Could you check a few things on this model? Use its own coordinates, in mm. A direction names the side the tool comes from. Give positions to 0.01 mm unless a question says otherwise; leave off trailing zeros. Loops run counter-clockwise (first coordinate to the right, second up) from the corner with the lowest first, then second, coordinate; pieces in that order, holes last. Notation, with made-up numbers: (-40, 44) -> (13, 44) arc R28 ccw to (13, 83) -> close; hole circle Ø8 at (88, -9). An arc over 180 degrees is marked (long way). Write item = value, one per line. Start each with the question number.
1) I want a section at A-A (z = 2.5). List the corners of the cut face in (x, y) for me, and give its area (3 significant figures).
2) I want a section at B-B (y = 13.5). List the corners of the cut face in (x, z) for me.
3) On a 3-axis mill with a long thin cutter (end or side, diameter ignored), from which of +Z, -Z, +X, -X, +Y, -Y can I reach the whole of each face in a straight line? I mean faces 1 (the face through (3, 4, 2)), 2 (the face through (-0.434, 10.793, 4.452)), 3 (the face through (-4.815, 1.215, 0.075)), 4 (the face through (-3, 4, 2)), 5 (the face through (-4.8, 1.1, 2.5)). Say none if no direction works.
4) I need wall thicknesses on probe 1 along X at (y, z) = (10.75, 2.45); probe 2 along X at (y, z) = (4.75, 2.3); probe 3 along Y at (x, z) = (-2.75, 2.2). Which ranges of each line are inside material? Lowest first, please. Write a range as from..to.
5) I'm going to push flat-ended pins straight in: pin 1 Ø1 at (y, z) = (4.5, 3.5) entering from +X; pin 2 Ø2 at (y, z) = (8.5, 3) entering from -X; pin 3 Ø0.8 at (x, z) = (5, 3.5) entering from +Y. Where does each tip first touch, or does it pass through?
from build123d import *

# Parameters (mm, degrees)
ESTRUSIONE_ESTRUSIONE1_DEPTH = 5
RACCORDO1_R                  = 0.25
SCHIZZO7_R                   = 2
ESTRUSIONE_ESTRUSIONE3_DEPTH = 12
SMUSSO1_SIZE                 = 0.25


with BuildPart() as part:
    # Schizzo1 → Estrusione-Estrusione1 (new body)
    with BuildSketch(Plane.XY):
        Polygon((3.7, 0), (-3.7, 0), (-6, 2.3), (-6, 3.3), (-3, 3.3), (-3, 5), (3, 5), (3, 3.3), (6, 3.3), (6, 2.3), align=None)
    extrude(amount=ESTRUSIONE_ESTRUSIONE1_DEPTH)

    # Raccordo1
    raccordo1_edges = [part.edges().sort_by_distance(p)[0] for p in [
        (-6, 2.8, 0),
        (-4.5, 3.3, 0),
        (-3, 4.15, 0),
        (0, 5, 0),
        (3, 4.15, 0),
        (4.5, 3.3, 0),
        (6, 2.8, 0),
        (4.85, 1.15, 5),
        (4.85, 1.15, 0),
        (0, 0, 0),
        (-4.85, 1.15, 0),
        (6, 2.8, 5),
        (-6, 2.3, 2.5),
        (-6, 3.3, 2.5),
        (-3, 3.3, 2.5),
        (-3, 5, 2.5),
        (3, 5, 2.5),
        (3, 3.3, 2.5),
        (-3.7, 0, 2.5),
        (4.5, 3.3, 5),
        (3, 4.15, 5),
        (0, 5, 5),
        (-3, 4.15, 5),
        (-4.5, 3.3, 5),
        (-6, 2.8, 5),
        (-4.85, 1.15, 5),
        (0, 0, 5),
    ]]
    fillet(raccordo1_edges, radius=RACCORDO1_R)

    # Schizzo7 → Estrusione-Estrusione3 (add)
    with BuildSketch(Plane(origin=(0, 5, 0), x_dir=(1, 0, 0), z_dir=(0, 1, 0))):
        with Locations((0, -2.5)):
            Circle(SCHIZZO7_R)
    extrude(amount=ESTRUSIONE_ESTRUSIONE3_DEPTH)

    # Smusso1
    smusso1_edges = [part.edges().sort_by_distance(p)[0] for p in [
        (-2, 17, 2.5),
    ]]
    chamfer(smusso1_edges, length=SMUSSO1_SIZE)

    # Schizzo8 → Rivoluzione2 (revolve)
    with BuildSketch(Plane.XY.offset(1.25)):
        Polygon((-4.5, 3.3), (-4.5, 3.55), (-4.75, 3.3), align=None)
    rivoluzione2 = revolve(axis=Axis((-4.5, 3.3, 1.25), (0, 1, 0)))

    # Specchia3: Rivoluzione2 across plane
    add(rivoluzione2.mirror(Plane(origin=(0, 0, 0), x_dir=(0, 0, 1), z_dir=(1, 0, 0))))

    # Specchia4: Rivoluzione2 across plane
    add(rivoluzione2.mirror(Plane.XY.offset(2.5)))

    # Specchia4 copy 1 sketch → Specchia4 copy 1 (revolve)
    with BuildSketch(Plane(origin=(0, 0, 3.75), x_dir=(-1, 0, 0), z_dir=(0, 0, -1))):
        Polygon((-4.5, 3.3), (-4.5, 3.55), (-4.75, 3.3), align=None)
    revolve(axis=Axis((4.5, 3.3, 3.75), (0, 1, 0)))


solid = part.part
Answer list:
q1.outline = (-6, 2.4) arc R0.25 ccw to (-5.93, 2.23) -> (-3.77, 0.07) arc R0.25 ccw to (-3.6, 0) -> (3.7, 0) -> (6, 2.3) -> (6, 3.3) -> (3.25, 3.3) arc R0.25 cw to (3, 3.55) -> (3, 4.75) arc R0.25 ccw to (2.75, 5) -> (2, 5) -> (2, 16.75) -> (1.75, 17) -> (-1.75, 17) -> (-2, 16.75) -> (-2, 5) -> (-2.75, 5) arc R0.25 ccw to (-3, 4.75) -> (-3, 3.55) arc R0.25 cw to (-3.25, 3.3) -> (-5.75, 3.3) arc R0.25 ccw to (-6, 3.05) -> close
q1.area = 92.4 mm^2
q2.outline = circle Ø4 at (0, 2.5)
q3.face_1 = +Z, -Z, +X, +Y
q3.face_2 = +Y
q3.face_3 = -Z, -X, -Y
q3.face_4 = +Z, -Z, -X, +Y
q3.face_5 = +Z, -Z, -X, -Y
q4.probe_1 = -2..2
q4.probe_2 = -3..3
q4.probe_3 = 0..5
q5.pin_1 = 3
q5.pin_2 = -2
q5.pin_3 = 3.39
